Geometry: final body of the model. Coordinates: model frame, mm. Face numbers are marked on the shaded views. A direction names the side the tool comes from. Coordinates: 2 decimals unless noted, no trailing zeros. Loops run counter-clockwise (first coordinate to the right, second up) from the corner with the lowest first, then second, coordinate; pieces in that order, holes last. Notation, with made-up numbers: (44.25, -33.5) - (68.25, -33.5) arc R16 ccw to (68.25, -27.5) - close; hole circle Ø6 at (80.5, 51). An arc over 180 degrees is marked (long way). Put each result on its own line as item: value. Start each with the question number.
1) Section A-A on x = 3.5. Output: boundary loops of the cut face in (y, z).
2) Contact query for a flat-ended pin moving along its axis: pin 1 Ø0.8 at (x, z) = (-4, -5) entering from +Y. Output: stop coordinate, or through.
3) Section B-B on z = -8.5. Output: boundary loops of the cut face in (x, y), and give its area (3 significant figures).
4) Section D-D on y = 1.9. Output: boundary loops of the cut face in (x, z).
5) Reachability of the marked faces 1, 2, 3 and 4 from +Z, -Z, +X, -X, +Y, -Y: full face, straight path, thin tool, end or side. Return the list, or none.
6) Draft query along Y for the marked faces 5, 6 and 7. Return one class per face: +Y half, -Y half, draft (parallel to the pull), parting line (faces both ways), or undercut.
7) Material intervals for line 1 along Y through (x, z) = (0, -2.25); line 2 along Y through (x, z) = (0, -5); line 3 along X through (y, z) = (4.55, -6.25), sorted ascending. Write a range as from..to.
8) Section C-C on x = -2. Output: boundary loops of the cut face in (y, z).
```python
from build123d import *

# Parameters (mm, degrees)
SKETCH_1_W          = 6
SKETCH_1_H          = 11.5
EXTRUDE_1_DEPTH     = 5
SKETCH_2_R          = 2.5
EXTRUDE_2_DEPTH     = 2.5
SKETCH_3_R          = 0.75
EXTRUDE_3_DEPTH     = 0.5
SKETCH_4_W          = 1
SKETCH_4_H          = 0.25
EXTRUDE_4_DEPTH     = 1.2
SKETCH_5_R          = 1.8
CUT_EXTRUDE_1_DEPTH = 15


with BuildPart() as part:
    # 草图1 → 凸台-拉伸1 (new body)
    with BuildSketch(Plane(origin=(0, 0, 0), x_dir=(1, 0, 0), z_dir=(0, 1, 0))):
        with Locations((0, 5.75)):
            Rectangle(SKETCH_1_W, SKETCH_1_H)
    extrude(amount=EXTRUDE_1_DEPTH)

    # 草图2 → 凸台-拉伸2 (add)
    with BuildSketch(Plane.XY):
        with Locations((0, 2.5)):
            Circle(SKETCH_2_R)
    extrude(amount=EXTRUDE_2_DEPTH)

    # 草图3 → 凸台-拉伸3 (add)
    with BuildSketch(Plane.XZ):
        with Locations((0, -2.5)):
            Circle(SKETCH_3_R)
        with Locations((0, -8.5)):
            Circle(SKETCH_3_R)
    extrude(amount=EXTRUDE_3_DEPTH)

    # 草图4 → 凸台-拉伸4 (add)
    with BuildSketch(Plane(origin=(3, 0, 0), x_dir=(0, 0, -1), z_dir=(1, 0, 0))):
        with Locations((1.8, 0.125)):
            Rectangle(SKETCH_4_W, SKETCH_4_H)
        with Locations((5, 0.125)):
            Rectangle(SKETCH_4_W, SKETCH_4_H)
        with Locations((8.5, 0.125)):
            Rectangle(SKETCH_4_W, SKETCH_4_H)
    extrude_4 = extrude(amount=EXTRUDE_4_DEPTH)

    # 镜向1: 凸台-拉伸4 across plane
    add(extrude_4.mirror(Plane(origin=(0, 0, 0), x_dir=(0, 0, 1), z_dir=(1, 0, 0))))

    # 草图5 → 切除-拉伸1 (cut, through all)
    with BuildSketch(Plane.XY.offset(2.5)):
        with Locations((0, 2.5)):
            Circle(SKETCH_5_R)
    extrude(amount=-CUT_EXTRUDE_1_DEPTH, mode=Mode.SUBTRACT)


solid = part.part
```
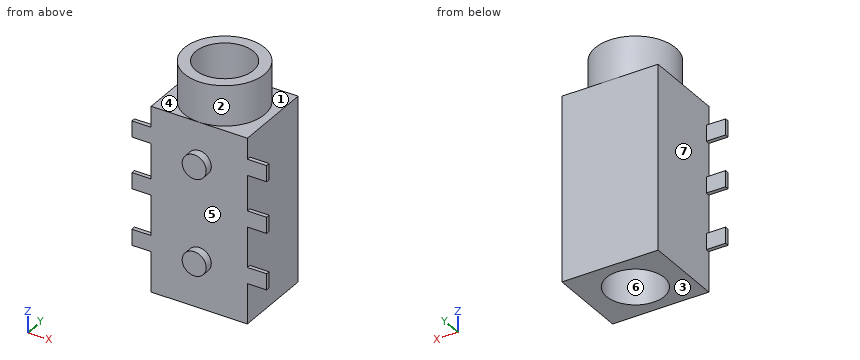
Answer block:
1. outline: (0, -9) - (0.25, -9) - (0.25, -8) - (0, -8) - close; (0, -5.5) - (0.25, -5.5) - (0.25, -4.5) - (0, -4.5) - close; (0, -2.3) - (0.25, -2.3) - (0.25, -1.3) - (0, -1.3) - close
2. pin 1: stops at y = 0.25
3. outline: (-4.2, 0) - (-0.75, 0) - (-0.75, -0.5) - (0.75, -0.5) - (0.75, 0) - (4.2, 0) - (4.2, 0.25) - (3, 0.25) - (3, 5) - (-3, 5) - (-3, 0.25) - (-4.2, 0.25) - close; hole circle Ø3.6 at (0, 2.5)
3. area: 21.2 mm²
4. outline: (-3, -11.5) - (-1.7, -11.5) - (-1.7, 2.5) - (-2.43, 2.5) - (-2.43, 0) - (-3, 0) - close; (1.7, -11.5) - (3, -11.5) - (3, 0) - (2.43, 0) - (2.43, 2.5) - (1.7, 2.5) - close
5. face 1: +Z, +X
5. face 2: +Z
5. face 3: -Z, +X, -X, +Y, -Y
5. face 4: +Z, -X
6. face 5: -Y half
6. face 6: undercut
6. face 7: draft
7. line 1: y = -0.5..0.7, 4.3..5
7. line 2: y = 0..0.7, 4.3..5
7. line 3: x = -3..3
8. outline: (0, -11.5) - (5, -11.5) - (5, 0) - (4, 0) - (4, 2.5) - (1, 2.5) - (1, 0) - (0, 0) - close
